Part model, mm, in its own coordinate system. A direction names the side the tool comes from. Coordinates: 2 decimals unless noted, no trailing zeros. Write each loop counter-clockwise with the first axis right and the second up, starting at its lowest first coordinate (ties: lowest second). Pieces come first, ordered by that corner, then holes. Notation, with made-up numbers: (45.25, -27) - (54.25, -27) arc R23 cw to (54.25, 11) - close; hole circle Ø6 at (15, -15.5). An arc over 180 degrees is marked (long way). Use one line per item in the form item = value. Start each with the question number.
from build123d import *

# Parameters (mm, degrees)
SKETCH1_W           = 14.986
SKETCH1_H           = 11.684
BOSS_EXTRUDE2_DEPTH = 8.89
SKETCH3_W           = 8.89
SKETCH3_H           = 11.684
BOSS_EXTRUDE4_DEPTH = 9.652
FILLET1_R           = 2.38
SKETCH4_R           = 1.905
BOSS_EXTRUDE5_DEPTH = 9.652
SKETCH5_R           = 0.889
CUT_EXTRUDE1_DEPTH  = 7.112


with BuildPart() as part:
    # Sketch1 → Boss-Extrude2 (new body)
    with BuildSketch(Plane(origin=(0, 0, 0), x_dir=(1, 0, 0), z_dir=(0, 1, 0))):
        with Locations((7.493, 5.842)):
            Rectangle(SKETCH1_W, SKETCH1_H)
    extrude(amount=BOSS_EXTRUDE2_DEPTH)

    # Sketch3 → Boss-Extrude4 (add)
    with BuildSketch(Plane.XZ):
        with Locations((-4.445, -5.842)):
            Rectangle(SKETCH3_W, SKETCH3_H)
    extrude(amount=-BOSS_EXTRUDE4_DEPTH)

    # Fillet1
    fillet1_edges = [part.edges().sort_by_distance(p)[0] for p in [
        (7.493, 8.89, 0),
        (7.493, 8.89, -11.684),
    ]]
    fillet(fillet1_edges, radius=FILLET1_R)

    # Sketch4 → Boss-Extrude5 (add)
    with BuildSketch(Plane.ZY.offset(8.89)):
        with Locations((-5.842, 4.826)):
            Circle(SKETCH4_R)
    extrude(amount=BOSS_EXTRUDE5_DEPTH)

    # Sketch5 → Cut-Extrude1 (cut)
    with BuildSketch(Plane.ZY.offset(8.89)):
        with Locations((-1.397, 4.826)):
            Circle(SKETCH5_R)
        with Locations((-10.287, 4.826)):
            Circle(SKETCH5_R)
    extrude(amount=-CUT_EXTRUDE1_DEPTH, mode=Mode.SUBTRACT)


solid = part.part
Q1. Slice it at C-C (y = 7.25). List the corners of the cut face in (x, z).
Q2. Slice it at D-D (x = 5). List the corners of the cut face in (y, z).
Q3. Slice it at A-A (z = -2.75). List the corners of the cut face in (x, y), plus the area to 3 significant figures.
Q4. Pin check, flat tips, straight feed: P1, Ø3, axis at y = 7, z = -1.5, coming from the -X side; P2, Ø3, axis at x = -12.5, z = -5, coming from the +Y side; P3, Ø0.9, axis at y = 5, z = -10.5, coming from the -X side. Stop position of each tip, or through.
Q5. Slice it at B-B (x = -6.5). List the corners of the cut face in (y, z), plus the area to 3 significant figures.
Q6. Which spindle directions (+Z, -Z, +X, -X, +Y, -Y) get a long thin tool onto all of the face, cutting with end or side? Do faces 1 (the cylindrical face through (7.6, 8.21, -10.97)), 2 (the flat face through (14.986, 4, -6)), 3 (the flat face through (0, 9.2, -5.9)), 4 (the cylindrical face through (-13.648, 5.398, -4.025)), 5 (the flat face through (7, 8.89, -6)). Say none if no direction does.
Q7. Mould opens along Y. For faces 6 (the flat face through (3, 0, -6)), 7 (the flat face through (-1.778, 5, -1)), 8 (the cylindrical face through (7.598, 8.211, -0.716)) say: released by +Y, released by -Y, zero draft, split by the parting line, or undercut.
Q8. Drill centre lines: probe 1 along X at (y, z) = (6.75, -7.25); probe 2 along X at (y, z) = (4, -1.5); probe 3 along Y at (x, z) = (4, -5.5). Where is each one in solid material? Low to high.
Solution:
q1.outline = (-8.89, -11.68) - (0, -11.68) - (0, -11.57) - (14.99, -11.57) - (14.99, -0.12) - (0, -0.12) - (0, 0) - (-8.89, 0) - close
q2.outline = (0, -11.68) - (6.51, -11.68) arc R2.38 ccw to (8.89, -9.3) - (8.89, -2.38) arc R2.38 ccw to (6.51, 0) - (0, 0) - close
q3.outline = (-8.89, 0) - (14.99, 0) - (14.99, 8.89) - (0, 8.89) - (0, 9.65) - (-8.89, 9.65) - close
q3.area = 219 mm2
q4.P1 = -8.89
q4.P2 = 6.73
q4.P3 = -1.78
q5.outline = (0, -11.68) - (9.65, -11.68) - (9.65, 0) - (0, 0) - close; hole circle Ø1.78 at (4.83, -10.29); hole circle Ø1.78 at (4.83, -1.4)
q5.area = 108 mm2
q6.face_1 = -Z, +X, +Y
q6.face_2 = +Z, -Z, +X, +Y, -Y
q6.face_3 = +X, +Y
q6.face_4 = -X
q6.face_5 = +Z, -Z, +X, +Y
q7.face_6 = released by -Y
q7.face_7 = undercut
q7.face_8 = released by +Y
q8.probe_1 = -8.89 to 14.99
q8.probe_2 = -1.78 to 14.99
q8.probe_3 = 0 to 8.89
